Here's how the part is built. I have some questions about the finished solid (model axes, mm). A direction names the side the tool comes from. Round coordinates to 2 decimals unless told otherwise and drop trailing zeros. Order: outer loops, then holes, each group sorted by start corner. A loop starts at its lowest first (then second) coordinate and runs counter-clockwise, first axis right, second up. Notation, with made-up numbers: M -12,28.25 L -7,28.25 A24 ccw -7,55.25 Z; hole C 6.5,19.5 d6. An arc over 180 degrees is marked long. Write item = value, one per line. Start each with the question number.
Item 1: For faces 1 (the face through (1, 7.9, -3)), 2 (the face through (2, 2, -6.5)), 3 (the face through (0, 4, -4)), which set-ups out of +Z, -Z, +X, -X, +Y, -Y let a thin tool reach every point of the face, with its end or its side?
Item 2: Please list where these lines run through material, in increasing order: L1, parallel to X at y = 8, z = -3.6; L2, parallel to X at y = 2, z = -4.25; L3, parallel to Z at x = 1.5, y = 4.
Item 3: I want a section at C-C, the plane z = -1. List the corners of the cut face in (x, y) for me, plus the area to 3 significant figures.
Item 4: I want a section at D-D, the plane y = 5.25. List the corners of the cut face in (x, z) for me.
Item 5: I'm going to push flat-ended pins straight in: P1, Ø1.5, axis at y = -1.5, z = -0.5, coming from the -X side; P2, Ø1, axis at x = 5, y = 2.5, coming from the +Z side; P3, Ø0.6, axis at x = 2.5, z = -3.5, coming from the +Y side. Where does each tip first touch, or does it pass through?
Item 6: I want a section at A-A, the plane y = -1.75. List the corners of the cut face in (x, z) for me.
Item 7: I want a section at B-B, the plane z = -2.75. State how many separate pieces and enclosed holes the cut face has, plus the area to 3 significant figures.
Item 8: We'd pull the mould along X, two halves only. Please class faces 4 (the face through (7, 4, -4)), 5 (the face through (6, 7.9, -3)), 6 (the face through (3.5, 8.4, -4.2)): pulls with the +X half, pulls with the -X half, needs draft (parallel to the pull), parting line crosses it, or undercut.
```python
from build123d import *

# Parameters (mm, degrees)
BOSS_EXTRUDE1_DEPTH         = 7
SKETCH2_R                   = 1.25
CUT_EXTRUDE1_DEPTH          = 0.5
SKETCH3_W                   = 3
SKETCH3_H                   = 4
CUT_EXTRUDE2_DEPTH          = 0.5
CUT_EXTRUDE2_TAPER          = 10
SKETCH4_R                   = 1
CUT_EXTRUDE3_DEPTH          = 6
SKETCH6_R                   = 0.45
BOSS_EXTRUDE3_DEPTH         = 3.8
CHAMFER1_SIZE               = 1
CHAMFER1_SIZE2              = 0.371896666
EXTRUDE_THIN1_DEPTH         = 0.75
SKETCH8_W                   = 0.25
SKETCH8_H                   = 2.158330758
SKETCH8_W_2                 = 1.874325027
SKETCH8_H_2                 = 0.25
CUT_EXTRUDE_THIN1_DEPTH     = 0.25
LPATTERN1_COUNT             = 2
LPATTERN1_PITCH             = 3.5
CHAMFER1_OF_LPATTERN1_SIZE2 = 0.371896666
CHAMFER1_OF_LPATTERN1_SIZE  = 1


with BuildPart() as part:
    # Sketch1 → Boss-Extrude1 (new body)
    with BuildSketch(Plane(origin=(0, 0, 0), x_dir=(0, 0, -1), z_dir=(1, 0, 0))):
        Polygon((0, 5), (1.5, 8.4), (7, 8.4), (7, 0), (0, 0), align=None)
    extrude(amount=BOSS_EXTRUDE1_DEPTH)

    # Sketch2 → Cut-Extrude1 (cut)
    with BuildSketch(Plane(origin=(0, 8.4, 0), x_dir=(1, 0, 0), z_dir=(0, 1, 0))):
        with Locations((1.75, 3.6)):
            Circle(SKETCH2_R)
    cut_extrude1 = extrude(amount=-CUT_EXTRUDE1_DEPTH, mode=Mode.SUBTRACT)

    # Sketch3 → Cut-Extrude2 (cut)
    with BuildSketch(Plane.XY):
        with Locations((1.75, 2.5)):
            Rectangle(SKETCH3_W, SKETCH3_H)
    cut_extrude2 = extrude(amount=-CUT_EXTRUDE2_DEPTH, taper=CUT_EXTRUDE2_TAPER, mode=Mode.SUBTRACT)

    # Sketch4 → Cut-Extrude3 (cut)
    with BuildSketch(Plane.XY.offset(-0.5)):
        with Locations((1.75, 2)):
            Circle(SKETCH4_R)
    cut_extrude3 = extrude(amount=-CUT_EXTRUDE3_DEPTH, mode=Mode.SUBTRACT)

    # Sketch6 → Boss-Extrude3 (add)
    with BuildSketch(Plane.XZ):
        with Locations((1.75, -3.6)):
            Circle(SKETCH6_R)
    boss_extrude3 = extrude(amount=BOSS_EXTRUDE3_DEPTH)

    # Chamfer1
    chamfer1_edges = [part.edges().sort_by_distance(p)[0] for p in [
        (1.3, -3.8, -3.6),
    ]]
    chamfer1_side = [part.faces().sort_by_distance(p)[0] for p in [
        (1.3, -1.9, -3.6),
    ]]
    chamfer(chamfer1_edges, length=CHAMFER1_SIZE, length2=CHAMFER1_SIZE2, reference=chamfer1_side[0])

    # Sketch7 → Extrude-Thin1 (add, symmetric)
    with BuildSketch(Plane(origin=(1.75, 0, 0), x_dir=(0, 0, -1), z_dir=(1, 0, 0))):
        Polygon((0.5, 3.678716588), (0.5, 2.743158903), (1.89970396, 1.832221158), (5.88813409, 1.438302133), (5.878305368, 1.338786324), (1.865601336, 1.735102771), (0.4, 2.688927019), (0.4, 3.678716588), align=None)
    extrude_thin1 = extrude(amount=EXTRUDE_THIN1_DEPTH, both=True)

    # Sketch8 → Cut-Extrude-Thin1 (cut, symmetric)
    with BuildSketch(Plane(origin=(0, 7.9, 0), x_dir=(1, 0, 0), z_dir=(0, 1, 0))):
        with Locations((1.75, 3.611637798)):
            Rectangle(SKETCH8_W, SKETCH8_H)
        with Locations((1.795143175, 3.611637798)):
            Rectangle(SKETCH8_W_2, SKETCH8_H_2)
    cut_extrude_thin1 = extrude(amount=CUT_EXTRUDE_THIN1_DEPTH, both=True, mode=Mode.SUBTRACT)

    # LPattern1: Cut-Extrude1, Cut-Extrude2, Cut-Extrude3, Boss-Extrude3, Extrude-Thin1, Cut-Extrude-Thin1 ×2
    with Locations(*[(i * LPATTERN1_PITCH, 0, 0) for i in range(1, LPATTERN1_COUNT)]):
        add(cut_extrude1, mode=Mode.SUBTRACT)
        add(cut_extrude2, mode=Mode.SUBTRACT)
        add(cut_extrude3, mode=Mode.SUBTRACT)
        add(boss_extrude3)
        add(extrude_thin1)
        add(cut_extrude_thin1, mode=Mode.SUBTRACT)

    # Chamfer1 of LPattern1
    chamfer1_of_lpattern1_edges = [part.edges().sort_by_distance(p)[0] for p in [
        (4.8, -3.8, -3.6),
    ]]
    chamfer(chamfer1_of_lpattern1_edges, length=CHAMFER1_OF_LPATTERN1_SIZE, length2=CHAMFER1_OF_LPATTERN1_SIZE2)


solid = part.part
```
Filled in:
q1.face_1 = +Y
q1.face_2 = none
q1.face_3 = +Z, -Z, -X, +Y, -Y
q2.L1 = 0 to 0.5, 3 to 4, 6.5 to 7
q2.L2 = 0 to 0.75, 2.75 to 4.25, 6.25 to 7
q2.L3 = -7 to -0.5
q3.outline = M 0,0 L 7,0 L 7,7.27 L 0,7.27 Z; M 1,2.3 L 2.5,2.3 L 2.5,2.42 L 1,2.42 Z; M 4.5,2.3 L 6,2.3 L 6,2.42 L 4.5,2.42 Z; hole C 1.75,2 d2; hole C 5.25,2 d2
q3.area = 44.9 mm^2
q4.outline = M 0,-7 L 7,-7 L 7,-0.11 L 0,-0.11 Z
q5.P1 = through
q5.P2 = -0.4
q5.P3 = 7.9
q6.outline = C 1.75,-3.6 d0.9; C 5.25,-3.6 d0.9
q7.separate_pieces = 3
q7.enclosed_holes = 2
q7.area = 50.9 mm^2
q8.face_4 = pulls with the +X half
q8.face_5 = undercut
q8.face_6 = needs draft
